from build123d import *

# Parameters (mm, degrees)
F1_DEPTH      = 2
F2_R          = 1.9
F3_DEPTH      = 88
F4_W          = 2
F4_H          = 30
F5_DEPTH      = 3
F6_DEPTH      = 2
F8_DEPTH      = 30.001
F9_W          = 10
F9_H          = 2.5
F10_DEPTH     = 92
F11_R         = 0.5
F12_W         = 10.5
F12_H         = 50
F13_DEPTH     = 5
F14_T1_DEPTH  = 10.5
F14_T3_DEPTH  = 10.5
F14_T8_DEPTH  = 34.9948974279
F14_T13_DEPTH = 34.9948974279
F14_T18_DEPTH = 35.5
F14_T23_DEPTH = 35.5


# Not quite as in the source:
# - a fillet or chamfer that OpenCascade refuses, or shapes differently, is made with other operations: its cross-section is extruded or revolved along the edge and cut away or added


with BuildPart() as f1:
    # F0 (on Top) → F1 (new body)
    with BuildSketch(Plane.XY):
        Polygon((0, 2), (0, 15), (-35, 15), (-35, -15), (0, -15), (0, -2), (-1, -2), (-1, 2), align=None)
    extrude(amount=F1_DEPTH)

    # F2 (on face) → F3 (join)
    with BuildSketch(Plane.XY.offset(2)):
        Polygon((-1, 2), (0, 2), (0, 10), (-10, 10), (-10, -10), (0, -10), (0, -2), (-1, -2), align=None)
        with Locations((-5, 0)):
            Circle(F2_R, mode=Mode.SUBTRACT)
    extrude(amount=F3_DEPTH)

    # F4 (on face) → F5 (join)
    with BuildSketch(Plane.XY.offset(2)):
        with Locations((-26, 0)):
            Rectangle(F4_W, F4_H)
        with Locations((-22, 0)):
            Rectangle(F4_W, F4_H)
    extrude(amount=F5_DEPTH)

    # F6 (add): a face of the model
    f6_faces = [f1.faces().sort_by_distance(p)[0] for p in [
        (-17.5650095602, 0, 0),
    ]]
    extrude(f6_faces, amount=F6_DEPTH)

    # F7 (on face) → F8 (cut, through all)
    with BuildSketch(Plane.XZ.offset(15)):
        Polygon((0, -2), (-35, 0), (-35, -2), align=None)
    extrude(amount=-F8_DEPTH, mode=Mode.SUBTRACT)

    # F9 (on face) → F10 (join)
    with BuildSketch(Plane.XY.offset(2)):
        with Locations((-5, 11.25)):
            Rectangle(F9_W, F9_H)
        with Locations((-5, -11.25)):
            Rectangle(F9_W, F9_H)
    extrude(amount=F10_DEPTH)

    # F11
    f11_edges = [f1.edges().sort_by_distance(p)[0] for p in [
        (-25, 0, 5),
        (-23, 0, 5),
        (-5, 10, 94),
        (-5, -10, 94),
    ]]
    fillet(f11_edges, radius=F11_R)

    # F12 (on face) → F13 (join)
    with BuildSketch(Plane.YZ):
        with Locations((7.25, 27)):
            Rectangle(F12_W, F12_H)
        with Locations((-7.25, 27)):
            Rectangle(F12_W, F12_H)
    extrude(amount=F13_DEPTH)

    # F14: fillet of radius 5 on 4 edges, made by hand

    # F14_s2 → F14_t1 (join)
    with BuildSketch(Plane.XZ.offset(2)):
        with BuildLine():
            ThreePointArc((0, -2), (1.7367018254, 0.8729833462), (4.8989794856, 2))
            Line((4.8989794856, 2), (0, 2))
            Line((0, 2), (0, -2))
        make_face()
        with BuildLine():
            ThreePointArc((0, 57), (1.4644660941, 53.4644660941), (5, 52))
            Line((5, 52), (0, 52))
            Line((0, 52), (0, 57))
        make_face()
    extrude(amount=F14_T1_DEPTH)

    # F14_s4 → F14_t3 (join)
    with BuildSketch(Plane.XZ.offset(-12.5)):
        with BuildLine():
            ThreePointArc((0, -2), (1.7367018254, 0.8729833462), (4.8989794856, 2))
            Line((4.8989794856, 2), (0, 2))
            Line((0, 2), (0, -2))
        make_face()
        with BuildLine():
            ThreePointArc((0, 57), (1.4644660941, 53.4644660941), (5, 52))
            Line((5, 52), (0, 52))
            Line((0, 52), (0, 57))
        make_face()
    extrude(amount=F14_T3_DEPTH)


with BuildPart() as f14_tool6:
    # F14_s7 → F14_t8 (new body)
    with BuildSketch(Plane.XZ.offset(24.7474487139)):
        with BuildLine():
            ThreePointArc((0, -2), (1.7367018254, 0.8729833462), (4.8989794856, 2))
            Line((4.8989794856, 2), (0, 2))
            Line((0, 2), (0, -2))
        make_face()
    extrude(amount=-F14_T8_DEPTH)

    split(bisect_by=Plane.XZ.offset(-2), keep=Keep.BOTTOM)


with BuildPart() as f1_1:
    add(f1.part)

    # F14_t5: union F14_tool6
    add(f14_tool6.part)


with BuildPart() as f14_tool11:
    # F14_s12 → F14_t13 (new body)
    with BuildSketch(Plane.XZ.offset(10.2474487139)):
        with BuildLine():
            ThreePointArc((0, -2), (1.7367018254, 0.8729833462), (4.8989794856, 2))
            Line((4.8989794856, 2), (0, 2))
            Line((0, 2), (0, -2))
        make_face()
    extrude(amount=-F14_T13_DEPTH)

    split(bisect_by=Plane.XZ.offset(2), keep=Keep.TOP)


with BuildPart() as f1_2:
    add(f1_1.part)

    # F14_t10: union F14_tool11
    add(f14_tool11.part)


with BuildPart() as f14_tool16:
    # F14_s17 → F14_t18 (new body)
    with BuildSketch(Plane.XZ.offset(-10.5)):
        with BuildLine():
            ThreePointArc((0, 57), (1.4644660941, 53.4644660941), (5, 52))
            Line((5, 52), (0, 52))
            Line((0, 52), (0, 57))
        make_face()
    extrude(amount=F14_T18_DEPTH)

    split(bisect_by=Plane.XZ.offset(-2), keep=Keep.BOTTOM)


with BuildPart() as f1_3:
    add(f1_2.part)

    # F14_t15: union F14_tool16
    add(f14_tool16.part)


with BuildPart() as f14_tool21:
    # F14_s22 → F14_t23 (new body)
    with BuildSketch(Plane.XZ.offset(-25)):
        with BuildLine():
            ThreePointArc((0, 57), (1.4644660941, 53.4644660941), (5, 52))
            Line((5, 52), (0, 52))
            Line((0, 52), (0, 57))
        make_face()
    extrude(amount=F14_T23_DEPTH)

    split(bisect_by=Plane.XZ.offset(2), keep=Keep.TOP)


with BuildPart() as f1_4:
    add(f1_3.part)

    # F14_t20: union F14_tool21
    add(f14_tool21.part)


solid = f1_4.part
Could you check a few things on this model? Use its own coordinates, in mm. A direction names the side the tool comes from. Give positions to 0.01 mm unless a question says otherwise; leave off trailing zeros. Order: outer loops, then holes, each group sorted by start corner. A loop starts at its lowest first (then second) coordinate and runs counter-clockwise, first axis right, second up. Notation, with made-up numbers: (-35, 35.5) -> (-9, 35.5) arc R33 cw to (-9, 74.5) -> close; hole circle Ø11 at (2, 19). An arc over 180 degrees is marked (long way). Return JSON: item names as keys, results as strings.
1. Imagine slicing it at B-B on y = 0. List the corners of the cut face in (x, z) for me, then the cut area to 3 significant figures.
Answer list:
{"outline": "(-35, 0) -> (-1, -1.94) -> (-1, 90) -> (-3.1, 90) -> (-3.1, 2) -> (-6.9, 2) -> (-6.9, 90) -> (-10, 90) -> (-10, 2) -> (-21, 2) -> (-21, 5) -> (-22.5, 5) arc R0.5 ccw to (-23, 4.5) -> (-23, 2) -> (-25, 2) -> (-25, 4.5) arc R0.5 ccw to (-25.5, 5) -> (-27, 5) -> (-27, 2) -> (-35, 2) -> close", "area": "571 mm2"}
2. Imagine slicing it at A-A on z = 82. List the corners of the cut face in (x, y) for me.
Answer list:
{"outline": "(-10, -12.5) -> (0, -12.5) -> (0, -2) -> (-1, -2) -> (-1, 2) -> (0, 2) -> (0, 12.5) -> (-10, 12.5) -> close; hole circle Ø3.8 at (-5, 0)"}
3. I need wall thicknesses on line 1 (Y direction, x = -5, z = 21.5); line 2 (Y direction, x = -5.5, z = 36); line 3 (X direction, y = -4, z = 6.5). Which ranges of each line are inside material? Lowest first, please. Write a range as from..to.
Answer list:
{"line 1": "y = -12.5..-1.9, 1.9..12.5", "line 2": "y = -12.5..-1.83, 1.83..12.5", "line 3": "x = -10..5"}
4. Imagine slicing it at C-C on x = -5. List the corners of the cut face in (y, z) for me.
Answer list:
{"outline": "(-15, -1.71) -> (15, -1.71) -> (15, 2) -> (12.5, 2) -> (12.5, 94) -> (10.5, 94) arc R0.5 ccw to (10, 93.5) -> (10, 90) -> (1.9, 90) -> (1.9, 2) -> (-1.9, 2) -> (-1.9, 90) -> (-10, 90) -> (-10, 93.5) arc R0.5 ccw to (-10.5, 94) -> (-12.5, 94) -> (-12.5, 2) -> (-15, 2) -> close"}
5. For pin 1 Ø11 at (x, y) = (-4, 0) entering from +Z; pin 2 Ø6.5 at (x, z) = (3, 65) entering from +Y; pin 3 Ø1.5 at (y, z) = (5.5, 4) entering from -X, each with a flat end and sliding along its axis, tell me the tip position at first contact or that it passes through.
Answer list:
{"pin 1": "stops at z = 90", "pin 2": "stops at y = 12.5", "pin 3": "stops at x = -27"}
6. Imagine slicing it at D-D on z = 23.5. List the corners of the cut face in (x, y) for me.
Answer list:
{"outline": "(-10, -12.5) -> (5, -12.5) -> (5, -2) -> (-1, -2) -> (-1, 2) -> (5, 2) -> (5, 12.5) -> (-10, 12.5) -> close; hole circle Ø3.8 at (-5, 0)"}
7. Thinking about a two-plate mould opening in X: for faces 4 (the flat face through (-5, 0, 2)), 5 (the flat face through (5, -7, 27)), 6 (the flat face through (-31, 0, 2)), which applies, pulls with the +X half, pulls with the -X half, needs draft (parallel to the pull), parting line crosses it, or undercut?
Answer list:
{"face 4": "undercut", "face 5": "pulls with the +X half", "face 6": "needs draft"}
8. On a 3-axis mill with a long thin cutter (end or side, diameter ignored), from which of +Z, -Z, +X, -X, +Y, -Y can I reach the whole of each face in a straight line? I mean faces 1 (the flat face through (-24, 0, 2)), 2 (the flat face through (0, 7, 75)), 3 (the flat face through (-7.3, 0.1, 90)). Say none if no direction works.
Answer list:
{"face 1": "+Z, +Y, -Y", "face 2": "+Z, +X, +Y, -Y", "face 3": "+Z, +X, -X"}
